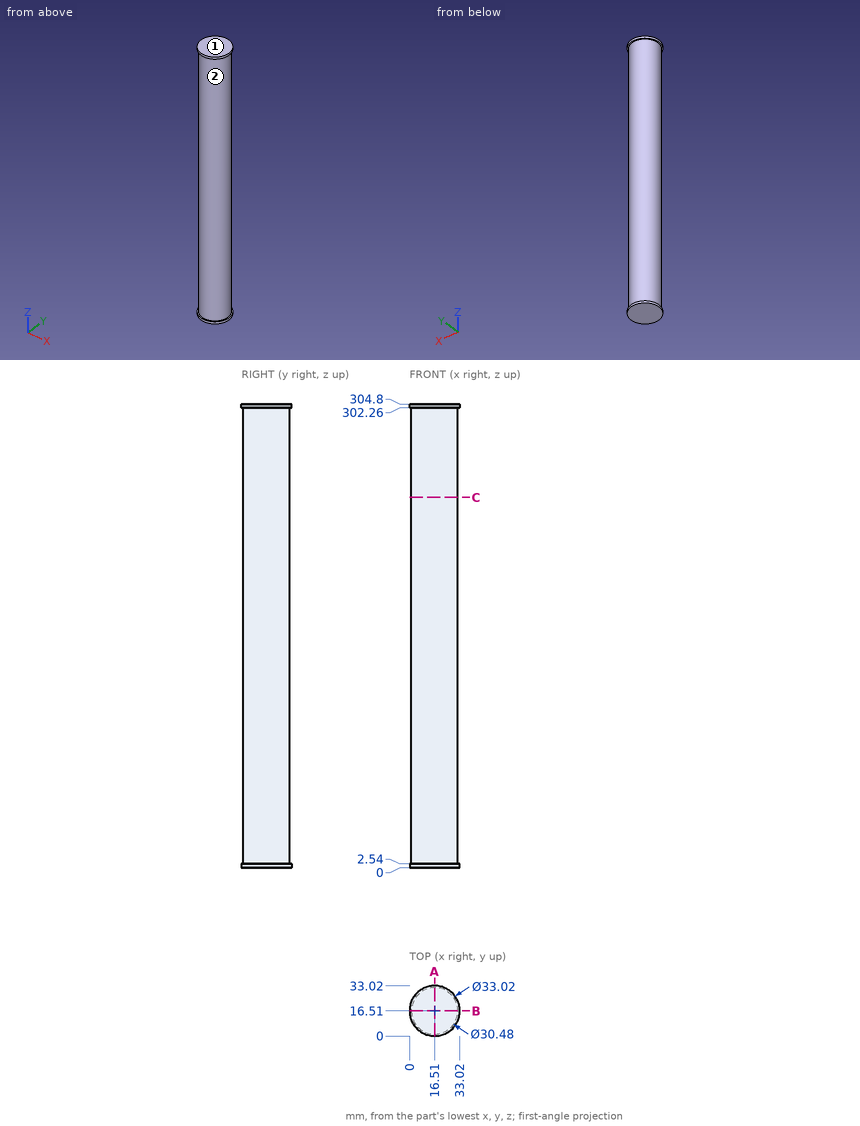
Here's the drawing with two shaded views (mm, measured from the low corner). I have some questions. A direction names the side the tool comes from. Round coordinates to 2 decimals unless told otherwise and drop trailing zeros. Loops run counter-clockwise (first coordinate to the right, second up) from the corner with the lowest first, then second, coordinate; pieces in that order, holes last. Notation, with made-up numbers: (47, 37.5) - (56, 37.5) arc R26 cw to (56, 62.5) - close; hole circle Ø10 at (-14, 89.25). An arc over 180 degrees is marked (long way). Use CSV: the item, a comma, the result in double quotes. Start each with the question number.
1) For pin 1 Ø12 at (y, z) = (15, 215.5) entering from -X; pin 2 Ø4 at (y, z) = (7, 41.5) entering from +X; pin 3 Ø4 at (x, z) = (10, 31) entering from +Y; pin 4 Ø2 at (x, y) = (22, 24.5) entering from -Z, each with a flat end and sliding along its axis, tell me the tip position at first contact or that it passes through.
2) If we section it at C-C on z = 243.5: Write out the boundary of the cut face in (x, y).
3) For the marked faces 1 and 2, which set-ups out of +Z, -Z, +X, -X, +Y, -Y let a thin tool reach every point of the face, with its end or its side?
4) If we section it at A-A on x = 16.51: Write out the boundary of the cut face in (y, z).
5) Please list where these lines run through material, in increasing order: probe 1 along Y at (x, z) = (17, 14.5); probe 2 along X at (y, z) = (9.5, 111.5); probe 3 along X at (y, z) = (4, 69). Write a range as [from, to].
Geometry results:
1,pin 1,"stops at x = 1.27"
1,pin 2,"stops at x = 29.77"
1,pin 3,"stops at y = 31.07"
1,pin 4,"stops at z = 0"
2,outline,"circle Ø30.48 at (16.51, 16.51)"
3,face 1,"+Z, +X, -X, +Y, -Y"
3,face 2,"none"
4,outline,"(0, 0) - (33.02, 0) - (33.02, 2.54) - (31.75, 2.54) - (31.75, 302.26) - (33.02, 302.26) - (33.02, 304.8) - (0, 304.8) - (0, 302.26) - (1.27, 302.26) - (1.27, 2.54) - (0, 2.54) - close"
5,probe 1,"y = [1.28, 31.74]"
5,probe 2,"x = [2.98, 30.04]"
5,probe 3,"x = [7.81, 25.21]"
